from build123d import *

# Parameters (mm, degrees)
SKETCH1_W           = 120
SKETCH1_H           = 60
BOSS_EXTRUDE1_DEPTH = 2.5
FILLET1_R           = 10
BOSS_EXTRUDE2_DEPTH = 30
LPATTERN1_COUNT     = 2
LPATTERN1_PITCH     = 60
SKETCH3_R           = 3
CUT_EXTRUDE1_DEPTH  = 72.3539808
CHAMFER1_SIZE       = 1


with BuildPart() as part:
    # Sketch1 → Boss-Extrude1 (new body)
    with BuildSketch(Plane(origin=(0, 0, 0), x_dir=(1, 0, 0), z_dir=(0, 1, 0))):
        Rectangle(SKETCH1_W, SKETCH1_H)
    extrude(amount=BOSS_EXTRUDE1_DEPTH)

    # Fillet1
    fillet1_edges = [part.edges().sort_by_distance(p)[0] for p in [
        (-60, 1.25, -30),
        (60, 1.25, -30),
    ]]
    fillet(fillet1_edges, radius=FILLET1_R)

    # Sketch3 → Cut-Extrude1 (cut, through all)
    with BuildSketch(Plane(origin=(0, 2.5, 0), x_dir=(1, 0, 0), z_dir=(0, 1, 0))):
        with Locations(Location((40, -10, 0), (0, 0, 270))):
            Circle(SKETCH3_R)
        with Locations(Location((0, 15, 0), (0, 0, 270))):
            Circle(SKETCH3_R)
        with Locations(Location((-40, -10, 0), (0, 0, 270))):
            Circle(SKETCH3_R)
    extrude(amount=-CUT_EXTRUDE1_DEPTH, mode=Mode.SUBTRACT)

    # Chamfer1
    chamfer1_edges = [part.edges().sort_by_distance(p)[0] for p in [
        (40, 2.5, 7),
        (0, 2.5, -18),
        (-40, 2.5, 7),
    ]]
    chamfer(chamfer1_edges, length=CHAMFER1_SIZE)


with BuildPart() as body_2:
    # Sketch2 → Boss-Extrude2 (new body)
    with BuildSketch(Plane(origin=(60, 0, 0), x_dir=(0, 0, -1), z_dir=(1, 0, 0))):
        with BuildLine():
            Line((-30, 2.5), (-30, -0.25))
            Line((-30, -0.25), (-30.7, -0.25))
            ThreePointArc((-30.7, -0.25), (-30.927169701, -0.304585668), (-31.104738562, -0.456424292))
            ThreePointArc((-31.104738562, -0.456424292), (-38.311548677, 2.389996547), (-30.625, 3.368358986))
            Line((-30.625, 3.368358986), (-32.325, 3.368358986))
            ThreePointArc((-32.325, 3.368358986), (-36.717094098, 1.109876278), (-31.842676994, 1.904415516))
            ThreePointArc((-31.842676994, 1.904415516), (-31.670115132, 2.325380148), (-31.25, 2.5))
            Line((-31.25, 2.5), (-30, 2.5))
        make_face()
    extrude(amount=-BOSS_EXTRUDE2_DEPTH)


with BuildPart() as lpattern1_1:
    # LPattern1: pattern copy
    add(body_2.part.moved(Location(Vector(-1, 0, 0) * (1 * LPATTERN1_PITCH))))

    # Combine1: union body 2, part
    add(body_2.part)
    add(part.part)


solid = lpattern1_1.part
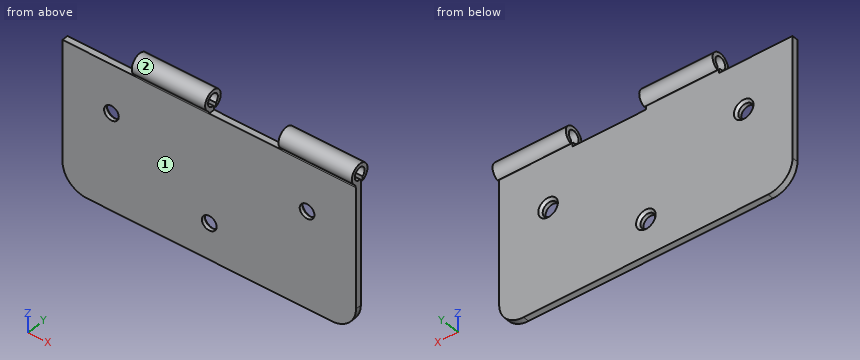
Can you work these out from the model? Positions are in its coordinate system, mm. Face numbers are marked on the shaded views. A direction names the side the tool comes from. Give positions to 0.01 mm unless a question says otherwise; leave off trailing zeros. Order: outer loops, then holes, each group sorted by start corner. A loop starts at its lowest first (then second) coordinate and runs counter-clockwise, first axis right, second up. Notation, with made-up numbers: M -31,24 L -27,24 A13 cw -27,45 Z; hole C 4.25,-13.5 d5. An arc over 180 degrees is marked long. Use one line per item in the form item = value.
Item 1: If we section it at C-C, the plane x = -25: Write out the boundary of the cut face in (y, z) (3 decimals), and give its area (3 significant figures).
Values follow:
outline = M -0.456,31.105 A0.5 cw -0.25,30.7 L -0.25,30 L 0,30 L 0,-30 L 2.5,-30 L 2.5,31.25 A0.593 ccw 1.904,31.843 A2.5 cw long 3.368,32.325 L 3.368,30.625 A4 ccw long Z
area = 181 mm^2
Item 2: If we section it at D-D, the plane x = -52: Write out the boundary of the cut face in (y, z).
Values follow:
outline = M 0,-29.8 L 2.5,-29.8 L 2.5,30 L 0,30 Z
Item 3: Will these pins go through, and if not, where does the flat tip stop? pin 1 Ø2 at (x, y) = (-43.5, 1) entering from +Z; pin 2 Ø18.5 at (x, z) = (25.5, -12) entering from +Y; pin 3 Ø1.9 at (x, z) = (39, 31.5) entering from -Y.
Values follow:
pin_1 = 30
pin_2 = 2.5
pin_3 = -1.63
Item 4: For the marked faces 1 and 2, which set-ups out of +Z, -Z, +X, -X, +Y, -Y let a thin tool reach every point of the face, with its end or its side?
Values follow:
face_1 = -Z, +X, -X, -Y
face_2 = +X, -X
Item 5: If I drill on line 1 along X through (y, z) = (0.65, 10); line 2 along Z through (x, y) = (45, 1.75); line 3 along Z through (x, y) = (23, 0.5), over which ranges is the centre line in solid material (lowest first)? Write a range as [from, to].
Values follow:
line_1 = [-60, -43], [-37, 37], [43, 60]
line_2 = [-30, 31.85], [36.84, 38.34]
line_3 = [-30, 30]
Item 6: If we section it at A-A, the plane z = -15: Write out the boundary of the cut face in (x, y), and give its area (3 significant figures).
Values follow:
outline = M -60,0 L -3,0 L -3,1.5 L -4,2.5 L -60,2.5 Z; M 3,0 L 60,0 L 60,2.5 L 4,2.5 L 3,1.5 Z
area = 284 mm^2
Item 7: If we section it at B-B, the plane x = -40: Write out the boundary of the cut face in (y, z).
Values follow:
outline = M 0,-30 L 2.5,-30 L 2.5,6 L 1.5,7 L 0,7 Z; M 0,13 L 1.5,13 L 2.5,14 L 2.5,30 L 0,30 Z
